Can you work these out from the drawing? Everything is in mm from the part's minimum corner. Give positions to 0.01 mm unless a question says otherwise; leave off trailing zeros. Order: outer loops, then holes, each group sorted by start corner. A loop starts at its lowest first (then second) coordinate and runs counter-clockwise, first axis right, second up. Notation, with made-up numbers: (63.25, 44) - (109.25, 44) arc R32 cw to (109.25, 75) - close; hole circle Ø1 at (89.25, -22). An arc over 180 degrees is marked (long way). One line per question, with ' | ' between items.
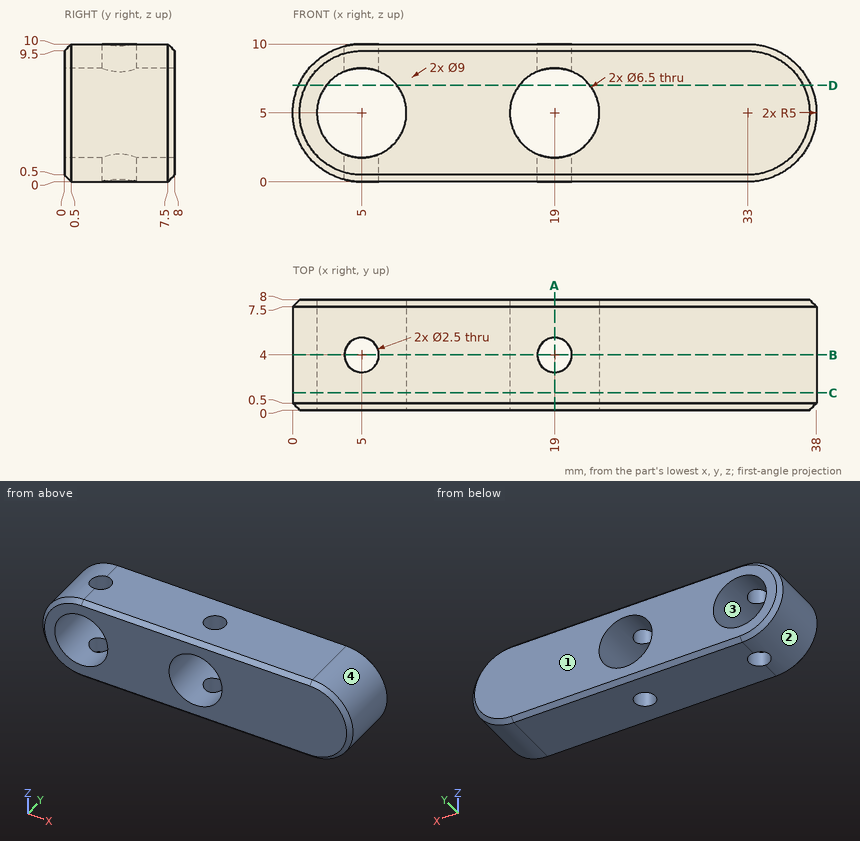
(1) Will these pins go through, and if not, where does the flat tip stop? pin 1 (4 mm diameter, centred on y = 7, z = 1.5, fed in from -X); pin 2 (2 mm diameter, centred on x = 19, y = 4, fed in from +Z).
Answer below:
pin 1: x = 0.23 | pin 2: through
(2) If we mould it in two halves opening along X, with no side actions, what happens to the marked faces 1, 2, 3 and 4? For each: released by +X, released by -X, zero draft, split by the parting line, or undercut.
Answer below:
face 1: zero draft | face 2: released by -X | face 3: undercut | face 4: released by +X
(3) Imagine slicing it at A-A (x = 19). List the corners of the cut face in (y, z) for me, and give its area (4 significant figures).
Answer below:
outline: (0, 0.5) - (0.5, 0) - (2.75, 0) - (2.75, 1.75) - (0, 1.75) - close; (0, 8.25) - (2.75, 8.25) - (2.75, 10) - (0.5, 10) - (0, 9.5) - close; (5.25, 0) - (7.5, 0) - (8, 0.5) - (8, 1.75) - (5.25, 1.75) - close; (5.25, 8.25) - (8, 8.25) - (8, 9.5) - (7.5, 10) - (5.25, 10) - close | area: 18.75 mm^2
(4) Imagine slicing it at C-C (y = 1.25). List the corners of the cut face in (x, z) for me, and give its area (3 significant figures).
Answer below:
outline: (5, 0) - (33, 0) arc R5 ccw to (33, 10) - (5, 10) arc R5 ccw to start; hole circle Ø6.5 at (5, 5); hole circle Ø6.5 at (19, 5) | area: 292 mm^2
(5) Imagine slicing it at B-B (y = 4). List the corners of the cut face in (x, z) for me, and give its area (3 significant figures).
Answer below:
outline: (3.75, 0.16) - (3.75, 2) arc R3.25 cw to (3.75, 8) - (3.75, 9.84) arc R5 ccw to start; (6.25, 0) - (17.75, 0) - (17.75, 2) arc R3.25 cw to (17.75, 8) - (17.75, 10) - (6.25, 10) - (6.25, 8) arc R3.25 cw to (6.25, 2) - close; (20.25, 0) - (33, 0) arc R5 ccw to (33, 10) - (20.25, 10) - (20.25, 8) arc R3.25 cw to (20.25, 2) - close | area: 274 mm^2
(6) If I drill on line 1 (X direction, y = 6.5, z = 5); line 2 (X direction, y = 2, z = 3.75); line 3 (Z direction, x = 22, y = 1), over which ranges is the centre line in solid material (lowest first)?
Answer below:
line 1: 0 to 1.75, 8.25 to 15.75, 22.25 to 38 | line 2: 0.16 to 2, 8 to 16, 22 to 37.84 | line 3: 0 to 3.75, 6.25 to 10
(7) Imagine slicing it at D-D (z = 7). Count the separate pieces of the cut face and the enclosed holes in it, and give its area (3 significant figures).
Answer below:
separate pieces: 3 | enclosed holes: 0 | area: 215 mm^2
